Build history of the part. All positions in model axes, mm. Face numbers are marked on the shaded views. A direction names the side the tool comes from. Round coordinates to 2 decimals unless told otherwise and drop trailing zeros. Write each loop counter-clockwise with the first axis right and the second up, starting at its lowest first coordinate (ties: lowest second). Pieces come first, ordered by that corner, then holes. Notation, with made-up numbers: (51.5, 7) - (104.5, 7) arc R15 cw to (104.5, 19) - close; hole circle Ø6 at (77, 86). An arc over 180 degrees is marked (long way). Answer as a JSON object with one key per item and string values. Group by question number.
Item 1: Probe line 1 (Y direction, x = 21, z = -14.5); line 2 (X direction, y = -12.5, z = -5.5); line 3 (Y direction, x = 13.25, z = -11). List the from-to ranges inside material, lowest first. Write a range as from..to.
Item 2: Two-plate mould, pull along Y, no slides. Class the marked faces 3, 4 and 5: +Y half, -Y half, draft (parallel to the pull), parting line (faces both ways), or undercut.
Item 3: Slice it at C-C, the plane y = -3.5. List the corners of the cut face in (x, z), then the cut area to 3 significant figures.
Item 4: Slice it at A-A, the plane z = -22. List the corners of the cut face in (x, y).
Item 5: Flat gauge pins, fed straight in: pin 1 (2.5 mm diameter, centred on x = 18.5, y = -5, fed in from +Z); pin 2 (6 mm diameter, centred on y = -9.5, z = -11, fed in from -X); pin 3 (6 mm diameter, centred on y = -7, z = -23, fed in from -X); pin 4 (3 mm diameter, centred on y = -10, z = -23, fed in from +X). Where does each tip first touch, or does it go through?
Item 6: Slice it at B-B, the plane x = 7. List the corners of the cut face in (y, z).
Item 7: Which spindle directions (+Z, -Z, +X, -X, +Y, -Y) get a long thin tool onto all of the face, cutting with end or side? Do the marked faces 1 and 2. Say none if no direction does.
Item 8: Slice it at D-D, the plane y = -12. List the corners of the cut face in (x, z), then the cut area to 3 significant figures.
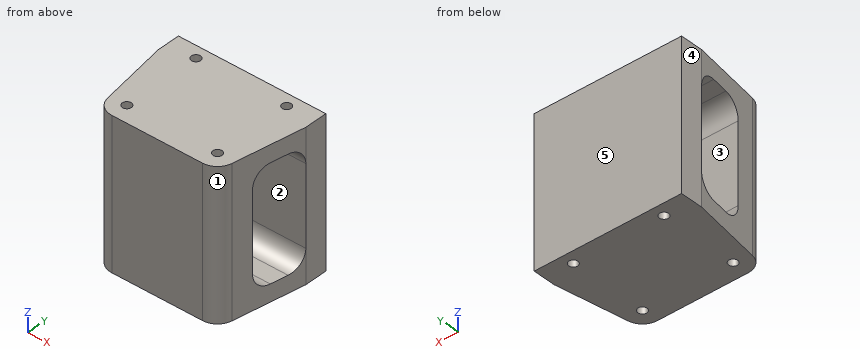
Autodesk Inventor part; units mm, degrees
ref_plane "YZ Plane" through (0, 0, 0) normal (1, 0, 0) x (0, 1, 0)
ref_plane "XZ Plane" through (0, 0, 0) normal (0, 1, 0) x (-1, 0, 0)
ref_plane "XY Plane" through (0, 0, 0) normal (0, 0, 1) x (1, 0, 0)
sketch "スケッチ3" plane through (0, 0, 0) normal (1, 0, 0) x (0, 1, 0)
  line L0 (0, 0) -> (4, 0)
  line L1 (4, 0) -> (4, -26)
  line L2 (4, -26) -> (0, -26)
  line L3 (0, -26) -> (0, 0)
  line L4 (4, 0) -> (0, 0)
  line L5 (0, 0) -> (0, -26)
  line L6 (0, -26) -> (4, -26)
  line L7 (4, -26) -> (4, 0)
  line L8 (0, 0) -> (-15, 0)
  line L9 (-15, 0) -> (-15, -26)
  line L10 (-15, -26) -> (0, -26)
  line L11 (0, -26) -> (0, 0)
  dimension "d3" = 26
  dimension "d4" = 4
  dimension "d49" = 15
extrude "押し出し2" add sketch "スケッチ3" along normal blind 26
sketch "スケッチ11" plane through (0, -15, 0) normal (0, 0, 1) x (1, 0, 0)
  circle A0 centre (5, 16.8437) radius 0.8
  circle A1 centre (21, 16.8437) radius 0.8
  point P0 (0, 15)
extrude "押し出し11" cut sketch "スケッチ11" against normal through all
sketch "スケッチ12" plane through (26, 0, 0) normal (1, 0, 0) x (0, 0, -1)
  line L0 (0, 4) -> (0, -15)
  line L1 (3, 0) -> (3, -9)
  line L2 (3, -9) -> (23, -9)
  line L3 (23, -9) -> (23, 0)
  line L4 (3, 0) -> (23, 0)
  line L5 (26, 4) -> (0, 4)
  line L6 (0, -15) -> (26, -15)
  point P0 (0, 0)
  point P1 (0, -0.1563)
  point P2 (13, 4)
  point P3 (13, 0)
  dimension "d62" = 3
  dimension "d63" = 6
extrude "押し出し12" cut sketch "スケッチ12" against normal through all
fillet "フィレット1" radius 3 4 edges at (13, 0, -23) (13, 0, -3) (13, -9, -23) (13, -9, -3)
sketch "スケッチ13" plane through (0, -15, 0) normal (0, 0, 1) x (1, 0, 0)
  line L0 (0, 15) -> (2.4503, 0)
  line L1 (0, 0) -> (26, 0)
  line L2 (26, 12) -> (26, 15)
  line L3 (26, 15) -> (23.5494, -0.0019)
  circle A0 centre (5, 3) radius 3
  circle A1 centre (21, 3) radius 3
  line L4 (0, 0) -> (26, 0)
  line L5 (0, 19) -> (26, 19)
  line L6 (13, 19) -> (13, 0)
  circle A2 centre (5, 3) radius 0.8
  circle A3 centre (21, 3) radius 0.8
  circle A4 centre (5, 16.8437) radius 0.8
  circle A5 centre (21, 16.8437) radius 0.8
  line L7 (0, 19) -> (0, 0)
  line L8 (0, 0) -> (26, 0)
  line L9 (26, 19) -> (26, 0)
  line L10 (0, 19) -> (26, 19)
  point P0 (5, 0)
  point P1 (2.0392, 2.5164)
  point P2 (23.9608, 2.5164)
  point P3 (21, 0)
  dimension "d64" = 16
  dimension "d65" = 6
  dimension "d66" = 1.6
  dimension "d67" = 1.6
extrude "押し出し13" cut sketch "スケッチ13" against normal through all contours L0 L1 L7 | A0 L1 L0 | A1 L3 L1 | L2 L9 L1 L3 | A2 | A3
properties part number "arm_middle"
Geometry says:
{
 "1": {"line 1": "y = -15..-12.8, -11.2..-9, 0..1.04, 2.64..4", "line 2": "x = 2.04..4.38, 5.62..20.38, 21.62..23.96", "line 3": "y = -15..-9, 0..4"},
 "2": {"face 3": "undercut", "face 4": "draft", "face 5": "+Y half"},
 "3": {"outline": "(0.57, -26) - (25.43, -26) - (25.43, -23) - (0.57, -23) - close; (0.57, -3) - (25.43, -3) - (25.43, 0) - (0.57, 0) - close", "area": "149 mm^2"},
 "4": {"outline": "(0, 0) - (0.12, -0.76) - (25.88, -0.76) - (26, 0) - (26, 4) - (0, 4) - close; (1.35, -8.24) - (2.04, -12.48) arc R3 ccw to (5, -15) - (21, -15) arc R3 ccw to (23.96, -12.48) - (24.65, -8.24) - close; hole circle Ø1.6 at (5, -12); hole circle Ø1.6 at (5, 1.84); hole circle Ø1.6 at (21, -12); hole circle Ø1.6 at (21, 1.84)"},
 "5": {"pin 1": "stops at z = 0", "pin 2": "stops at x = 1.47", "pin 3": "stops at x = 0.65", "pin 4": "stops at x = 24.61"},
 "6": {"outline": "(-15, -26) - (4, -26) - (4, 0) - (-15, 0) - close; hole (-9, -20) arc R3 ccw to (-6, -23) - (-3, -23) arc R3 ccw to (0, -20) - (0, -6) arc R3 ccw to (-3, -3) - (-6, -3) arc R3 ccw to (-9, -6) - close"},
 "7": {"face 1": "+Z, -Z, +X, -Y", "face 2": "+X, -X"},
 "8": {"outline": "(1.96, -26) - (4.2, -26) - (4.2, 0) - (1.96, 0) - close; (5.8, -26) - (20.2, -26) - (20.2, 0) - (5.8, 0) - close; (21.8, -26) - (24.04, -26) - (24.04, 0) - (21.8, 0) - close", "area": "491 mm^2"}
}
